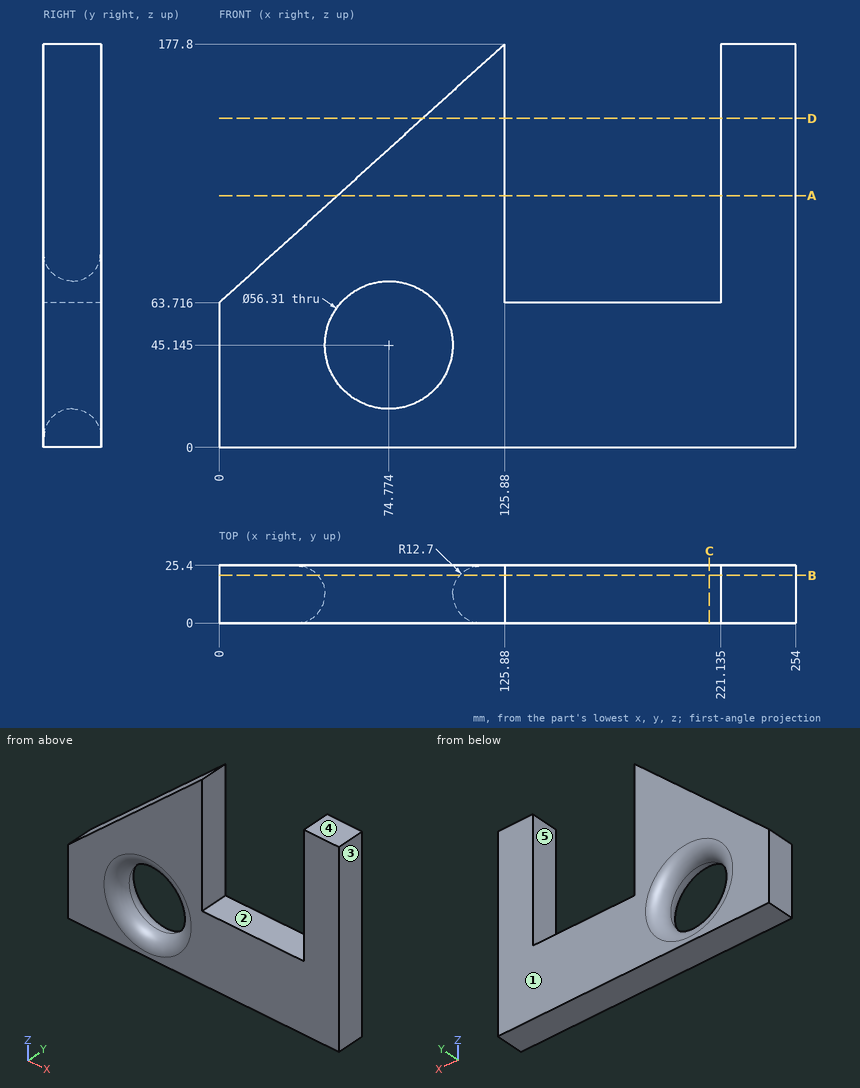
For this review, use the dimensioned drawing (mm, ordinates from the lowest corner) and the shaded views. A direction names the side the tool comes from. Round coordinates to 2 decimals unless told otherwise and drop trailing zeros. Write each loop counter-clockwise with the first axis right and the second up, starting at its lowest first coordinate (ties: lowest second). Pieces come first, ordered by that corner, then holes. Notation, with made-up numbers: M 63.25,47.25 L 106.25,47.25 A30 cw 106.25,69.25 Z; hole C -24.75,41.25 d1. An arc over 180 degrees is marked long. Answer as CSV lines item,"result". Start each with the question number.
Q1. Consider section D-D, the plane z = 145. Give the boundary of the cut face in (x, y) (1 decimal).
Q2. Consider section C-C, the plane x = 216. Give the boundary of the cut face in (y, z), then the cut area to 3 significant figures.
Q3. Tool access review of the marked faces 4 and 5: name each direction out of +Z, -Z, +X, -X, +Y, -Y from which nothing blocks a thin tool from reaching the whole face with its end or side.
Q4. The part is to be moulded in two halves that separate along X. For the marked faces 1, 2 and 3, say which applies: +X half, -X half, draft (parallel to the pull), parting line (faces both ways), or undercut.
Q5. Consider section A-A, the plane z = 111. Give the boundary of the cut face in (x, y) (1 decimal).
Q6. Clearance check with flat-ended pins moving along their axes: P1, Ø12, axis at x = 192, y = 14, coming from the +Z side; P2, Ø7.5, axis at y = 18, z = 95.5, coming from the -X side; P3, Ø1.5, axis at x = 114.5, y = 5, coming from the +Z side (1 decimal). State where each tip first meets the part, or that it passes through.
Q7. Consider section B-B, the plane y = 21. Give the boundary of the cut face in (x, z) (1 decimal).
Q8. Wall thickness on line 1 along X through (y, z) = (4.5, 94.5) (1 decimal); line 2 along X through (y, z) = (6.5, 82) (1 decimal); line 3 along Z through (x, y) = (151, 14.25): over which ranges is each line inside the solid? List them lowest first.
Result set:
1,outline,"M 89.7,0 L 125.9,0 L 125.9,25.4 L 89.7,25.4 Z; M 221.1,0 L 254,0 L 254,25.4 L 221.1,25.4 Z"
2,outline,"M 0,0 L 25.4,0 L 25.4,63.72 L 0,63.72 Z"
2,area,"1,620 mm²"
3,face 4,"+Z, +X, -X, +Y, -Y"
3,face 5,"+Z, +Y, -Y"
4,face 1,"draft"
4,face 2,"undercut"
4,face 3,"+X half"
5,outline,"M 52.2,0 L 125.9,0 L 125.9,25.4 L 52.2,25.4 Z; M 221.1,0 L 254,0 L 254,25.4 L 221.1,25.4 Z"
6,P1,"stops at z = 63.72"
6,P2,"stops at x = 30.93"
6,P3,"stops at z = 168.2"
7,outline,"M 0,0 L 254,0 L 254,177.8 L 221.1,177.8 L 221.1,63.7 L 125.9,63.7 L 125.9,177.8 L 0,63.7 Z; hole C 74.8,45.1 d62.5"
8,line 1,"x = 34 to 125.9, 221.1 to 254"
8,line 2,"x = 20.2 to 125.9, 221.1 to 254"
8,line 3,"z = 0 to 63.72"
